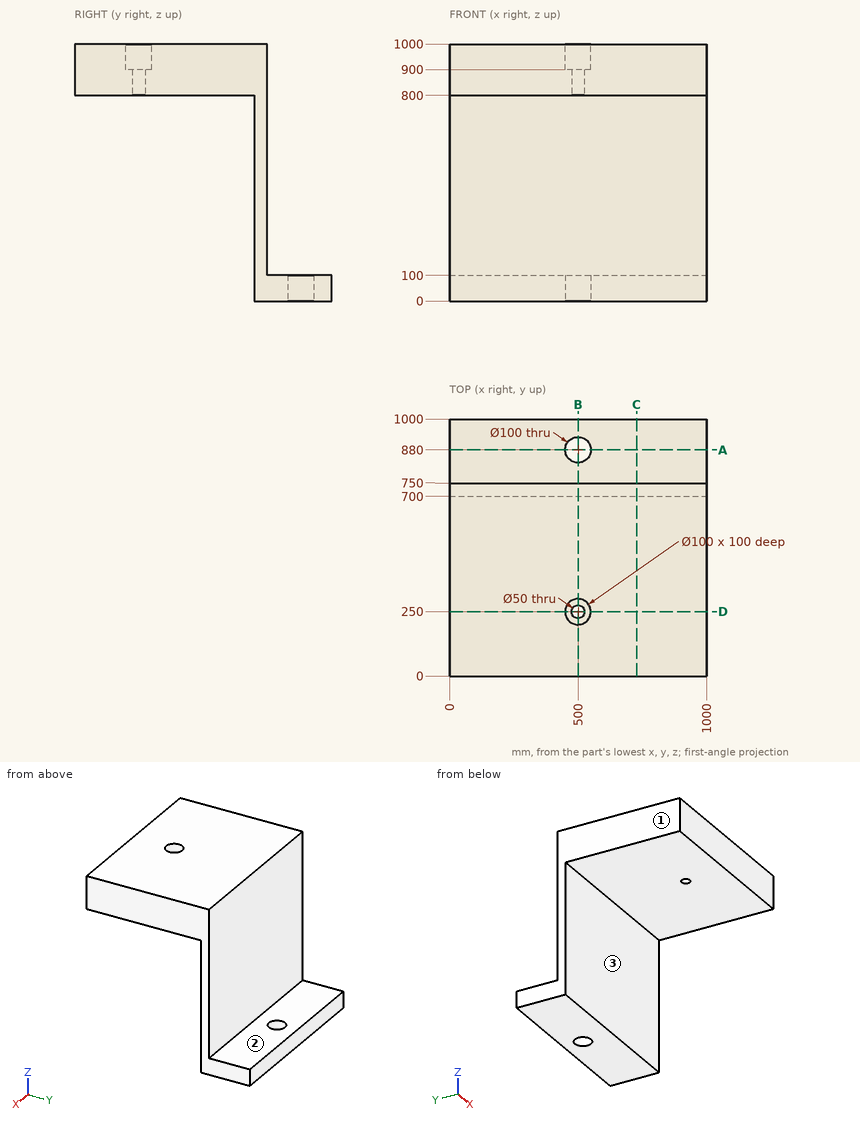
The figure shows three views and two pictorial views of one solid part (mm, origin at its lowest corner). Answer the questions. A direction names the side the tool comes from. Coordinates: 2 decimals unless noted, no trailing zeros. Loops run counter-clockwise (first coordinate to the right, second up) from the corner with the lowest first, then second, coordinate; pieces in that order, holes last. Notation, with made-up numbers: (4, 82.5) -> (21, 82.5) arc R17 cw to (21, 97.5) -> close; hole circle Ø2 at (66.25, 69.5). An arc over 180 degrees is marked (long way). Write item = value, one per line. Start each with the question number.
1) Straight lines are drawn through the part: line 1 (Y direction, x = 500, z = 939); line 2 (Y direction, x = 500, z = 61); line 3 (Y direction, x = 392, z = 895.5). For each, find the intervals that lie inside material, in ascending order. Write a range as from..to.
2) A cutting plane is placed at C-C (x = 728). Give the vertices of the cut face in (y, z).
3) A cutting plane is placed at D-D (y = 250). Give the vertices of the cut face in (x, z).
4) A cutting plane is placed at B-B (x = 500). Give the vertices of the cut face in (y, z).
5) A tool of negligible diameter and unlimited length cuts with its end or side. For the marked faces 1, 2 and 3, from which of +Z, -Z, +X, -X, +Y, -Y can it reach the whole face along a straight path? Write none if from no direction.
6) Given pin 1 Ø3 at (x, y) = (816.5, 860) entering from +Z; pin 2 Ø2 at (x, z) = (650.5, 305) entering from -Y; pin 3 Ø1.5 at (x, y) = (418.5, 318) entering from -Z, each flat-ended and moving along its own axis, determine where each tip first touches the part or whether it passes through.
7) A cutting plane is placed at A-A (y = 880). Give the vertices of the cut face in (x, z).
Responses:
q1.line_1 = 0..200, 300..750
q1.line_2 = 700..830, 930..1000
q1.line_3 = 0..750
q2.outline = (0, 800) -> (700, 800) -> (700, 0) -> (1000, 0) -> (1000, 100) -> (750, 100) -> (750, 1000) -> (0, 1000) -> close
q3.outline = (0, 800) -> (475, 800) -> (475, 900) -> (450, 900) -> (450, 1000) -> (0, 1000) -> close; (525, 800) -> (1000, 800) -> (1000, 1000) -> (550, 1000) -> (550, 900) -> (525, 900) -> close
q4.outline = (0, 800) -> (225, 800) -> (225, 900) -> (200, 900) -> (200, 1000) -> (0, 1000) -> close; (275, 800) -> (700, 800) -> (700, 0) -> (830, 0) -> (830, 100) -> (750, 100) -> (750, 1000) -> (300, 1000) -> (300, 900) -> (275, 900) -> close; (930, 0) -> (1000, 0) -> (1000, 100) -> (930, 100) -> close
q5.face_1 = +Z, -Z, -X, +Y, -Y
q5.face_2 = +Z, +X, -X, +Y
q5.face_3 = -Z, +X, -X, -Y
q6.pin_1 = 100
q6.pin_2 = 700
q6.pin_3 = 800
q7.outline = (0, 0) -> (450, 0) -> (450, 100) -> (0, 100) -> close; (550, 0) -> (1000, 0) -> (1000, 100) -> (550, 100) -> close
